from build123d import *

# Parameters (mm, degrees)
SKETCH_W        = 73
SKETCH_H        = 37
PAD_DEPTH       = 4
SKETCH001_W     = 4
SKETCH001_H     = 31
PAD001_DEPTH    = 25
SKETCH002_W     = 16
SKETCH002_H     = 5
PAD002_DEPTH    = 46
SKETCH003_W     = 16
SKETCH003_H     = 6
PAD003_DEPTH    = 14
SKETCH004_R     = 5.25
POCKET_DEPTH    = 6
CHAMFER_SIZE    = 28
CHAMFER001_SIZE = 28
CHAMFER002_SIZE = 10
SKETCH005_R     = 5
POCKET001_DEPTH = 5


with BuildPart() as part:
    # Sketch → Pad (new body)
    with BuildSketch(Plane.XY):
        Rectangle(SKETCH_W, SKETCH_H)
    extrude(amount=PAD_DEPTH)

    # Sketch001 (on Face6 of Pad) → Pad001 (join)
    with BuildSketch(Plane.XY.offset(4)):
        with Locations((-28.5, -3)):
            Rectangle(SKETCH001_W, SKETCH001_H)
        with Locations((28.5, -3)):
            Rectangle(SKETCH001_W, SKETCH001_H)
    extrude(amount=PAD001_DEPTH)

    # Sketch002 (on Face4 of Pad001) → Pad002 (join)
    with BuildSketch(Plane(origin=(0, 0, 0), x_dir=(1, 0, 0), z_dir=(0, 0, -1))):
        with Locations((0, 4)):
            Rectangle(SKETCH002_W, SKETCH002_H)
    extrude(amount=PAD002_DEPTH)

    # Sketch003 (on Face8 of Pad002) → Pad003 (join)
    with BuildSketch(Plane(origin=(0, -1.5, 0), x_dir=(-1, 0, 0), z_dir=(0, 1, 0))):
        with Locations((0, -43)):
            Rectangle(SKETCH003_W, SKETCH003_H)
    extrude(amount=PAD003_DEPTH)

    # Sketch004 (on Face25 of Pad003) → Pocket (cut)
    with BuildSketch(Plane(origin=(0, 0, -46), x_dir=(1, 0, 0), z_dir=(0, 0, -1))):
        with Locations((0, -6.5)):
            Circle(SKETCH004_R)
    extrude(amount=-POCKET_DEPTH, mode=Mode.SUBTRACT)

    # Chamfer
    chamfer_edges = [part.edges().sort_by_distance(p)[0] for p in [
        (8, -4, 0),
    ]]
    chamfer(chamfer_edges, length=CHAMFER_SIZE)

    # Chamfer001
    chamfer001_edges = [part.edges().sort_by_distance(p)[0] for p in [
        (-8, -4, 0),
    ]]
    chamfer(chamfer001_edges, length=CHAMFER001_SIZE)

    # Chamfer002
    chamfer002_edges = [part.edges().sort_by_distance(p)[0] for p in [
        (0, -6.5, 0),
    ]]
    chamfer(chamfer002_edges, length=CHAMFER002_SIZE)

    # Sketch005 (on Face1 of Chamfer002) → Pocket001 (cut)
    with BuildSketch(Plane(origin=(0, 0, 0), x_dir=(1, 0, 0), z_dir=(0, 0, -1))):
        with Locations((15, -6.5)):
            Circle(SKETCH005_R)
        with Locations((-15, -6.5)):
            Circle(SKETCH005_R)
    extrude(amount=-POCKET001_DEPTH, mode=Mode.SUBTRACT)


solid = part.part
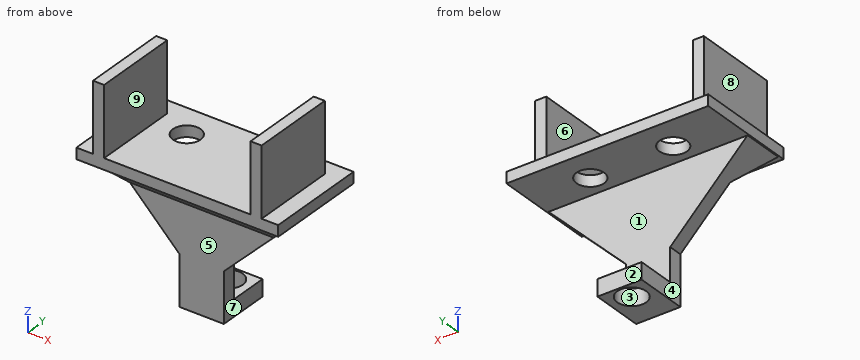
Could you check a few things on this model? Use its own coordinates, in mm. Face numbers are marked on the shaded views. A direction names the side the tool comes from. Give positions to 0.01 mm unless a question says otherwise; leave off trailing zeros. Write each loop counter-clockwise with the first axis right and the second up, starting at its lowest first coordinate (ties: lowest second). Pieces come first, ordered by that corner, then holes. Notation, with made-up numbers: (-17.75, 77.25) -> (22.25, 77.25) arc R33 ccw to (22.25, 109.25) -> close; hole circle Ø2 at (34, 15). An arc over 180 degrees is marked (long way). Write each question's results on one line, items separated by ' | '. Start each with the question number.
Q1. I'm going to push flat-ended pins straight in: pin 1 Ø12.5 at (y, z) = (1.5, 20) entering from +X; pin 2 Ø6 at (x, y) = (-24, 8.5) entering from -Z; pin 3 Ø12 at (y, z) = (-3.5, -32) entering from +X. Where does each tip first touch, or does it pass through?
Q2. Suppose I cut it at C-C, the plane y = 6.5. List the corners of the cut face in (x, z) for me.
Q3. Suppose I cut it at A-A, the plane x = 0. List the corners of the cut face in (y, z) for me.
Q4. I need wall thicknesses on probe 1 along X at (y, z) = (6.5, 2.4); probe 2 along X at (y, z) = (0, 22); probe 3 along Y at (x, z) = (-15, 1.6). Which ranges of each line are inside material? Lowest first, please.
Q5. Suppose I cut it at D-D, the plane x = 24. List the corners of the cut face in (y, z) for me, and give its area (3 significant figures).
Q6. Suppose I cut it at B-B, the plane z = 12. List the corners of the cut face in (x, y) for me, and give its area (3 significant figures).
Q7. We'd pull the mould along X, two halves only. Please class the marked faces 6, 7, 8 and 9: +X half, -X half, draft (parallel to the pull), parting line (faces both ways), or undercut.
Q8. Which directions (+Z, -Z, +X, -X, +Y, -Y) give clear straight access to the entire face, cutting with the end or side of a thin tool? Please do the marked faces 1, 2, 3, 4 and 5.
Outcome:
1) pin 1: x = 30.5 | pin 2: z = 0 | pin 3: x = 10
2) outline: (-36.5, 0) -> (-20, 0) -> (-20, 4) -> (-26.5, 4) -> (-26.5, 29) -> (-30.5, 29) -> (-30.5, 4) -> (-36.5, 4) -> close; (-10, 0) -> (10, 0) -> (10, 4) -> (-10, 4) -> close; (-8, -46) -> (-5.25, -46) -> (-5.25, -40) -> (-8, -40) -> close; (5.25, -46) -> (8, -46) -> (8, -40) -> (5.25, -40) -> close; (20, 0) -> (36.5, 0) -> (36.5, 4) -> (30.5, 4) -> (30.5, 29) -> (26.5, 29) -> (26.5, 4) -> (20, 4) -> close
3) outline: (-18.5, 0) -> (-16.5, 0) -> (-6.5, -10) -> (-6.5, -46) -> (1.25, -46) -> (1.25, -40) -> (-1.5, -40) -> (-1.5, 0) -> (18.5, 0) -> (18.5, 4) -> (-18.5, 4) -> close; (11.75, -46) -> (12.5, -46) -> (12.5, -40) -> (11.75, -40) -> close
4) probe 1: -36.5 to -20, -10 to 10, 20 to 36.5 | probe 2: -30.5 to -26.5, 26.5 to 30.5 | probe 3: -18.5 to 1.5, 11.5 to 18.5
5) outline: (-18.5, 0) -> (-16.5, 0) -> (-6.5, -10) -> (-6.5, -12) -> (-1.5, -12) -> (-1.5, 0) -> (18.5, 0) -> (18.5, 4) -> (-18.5, 4) -> close | area: 258 mm2
6) outline: (-30.5, -18.5) -> (-26.5, -18.5) -> (-26.5, 12.5) -> (-30.5, 12.5) -> close; (26.5, -18.5) -> (30.5, -18.5) -> (30.5, 12.5) -> (26.5, 12.5) -> close | area: 248 mm2
7) face 6: undercut | face 7: +X half | face 8: -X half | face 9: undercut
8) face 1: +X, -X, +Y | face 2: -Z, +X, -X, +Y | face 3: -Z | face 4: -Z, -X, +Y, -Y | face 5: -Z, +X, -X, -Y
